```python
from build123d import *

# Parameters (mm, degrees)
SKETCH2_R          = 2
CUT_EXTRUDE1_DEPTH = 20.646882704


with BuildPart() as part:
    # Sketch1 → Revolve1 (revolve)
    with BuildSketch(Plane.XY, mode=Mode.PRIVATE) as revolve1_sk:
        Polygon((-4, 0), (-11, 0), (-11, 3), (-5, 3), (-5, 15), (-4, 15), align=None)
    revolve(revolve1_sk.sketch.rotate(Axis((0, -177.201778129, 0), (0, 1, 0)), 180), axis=Axis((0, -177.201778129, 0), (0, 1, 0)))

    # Sketch2 → Cut-Extrude1 (cut, through all)
    with BuildSketch(Plane(origin=(0, 3, 0), x_dir=(1, 0, 0), z_dir=(0, 1, 0))):
        with Locations(Location((0, 8, 0), (0, 0, 180))):
            Circle(SKETCH2_R)
        with Locations(Location((8, 0, 0), (0, 0, 180))):
            Circle(SKETCH2_R)
        with Locations(Location((0, -8, 0), (0, 0, 180))):
            Circle(SKETCH2_R)
        with Locations(Location((-8, 0, 0), (0, 0, 180))):
            Circle(SKETCH2_R)
    extrude(amount=-CUT_EXTRUDE1_DEPTH, mode=Mode.SUBTRACT)


solid = part.part
```
Source: CAD feature listing. Evaluate the final solid. Frame: model axes, mm. A direction names the side the tool comes from. Coordinates: 2 decimals unless noted, no trailing zeros. Order: outer loops, then holes, each group sorted by start corner. A loop starts at its lowest first (then second) coordinate and runs counter-clockwise, first axis right, second up. Notation, with made-up numbers: (-29.75, 81) - (-15.75, 81) arc R15 cw to (-15.75, 108) - close; hole circle Ø3 at (-4.75, 5). An arc over 180 degrees is marked (long way). One line per item, written item: value.
1) Cut plane D-D on z = -8. Output: boundary loops of the cut face in (x, y), plus the area to 3 significant figures.
Computed values:
outline: (-7.55, 0) - (-2, 0) - (-2, 3) - (-7.55, 3) - close; (2, 0) - (7.55, 0) - (7.55, 3) - (2, 3) - close
area: 33.3 mm^2
2) Contact query for flat-ended pins moving along their axis: pin 1 (4 mm diameter, centred on x = 6, z = -4, fed in from -Y); pin 2 (5 mm diameter, centred on x = -8, z = 0, fed in from +Y); pin 3 (5 mm diameter, centred on x = -3.5, y = 3, fed in from +Z); pin 4 (8 mm diameter, centred on x = -7.5, y = 9, fed in from -Z). Output: stop coordinate, or through.
Computed values:
pin 1: stops at y = 0
pin 2: stops at y = 3
pin 3: stops at z = 10.95
pin 4: stops at z = -3.57
3) Cut plane C-C on y = 13. Output: boundary loops of the cut face in (x, z).
Computed values:
outline: circle Ø10 at (0, 0); hole circle Ø8 at (0, 0)
4) Reachability of faces 4 (the face through (2, 3, 5)), 5 (the face through (-2.38, 1.52, 10.74)) from +Z, -Z, +X, -X, +Y, -Y: full face, straight path, thin tool, end or side. Return the list, or none.
Computed values:
face 4: +Y
face 5: +Y, -Y
5) Ray query, line 1 (X direction, y = 1.75, z = 0.75); line 2 (Y direction, x = -3, z = -7.5); line 3 (Z direction, x = 1.5, y = 0.5). Return the intervals inside material, ascending. Write a range as [from, to].
Computed values:
line 1: x = [-10.97, -9.85], [-6.15, -3.93], [3.93, 6.15], [9.85, 10.97]
line 2: y = [0, 3]
line 3: z = [-10.9, -9.32], [-6.68, -3.71], [3.71, 6.68], [9.32, 10.9]
6) Cut plane A-A on z = 3. Output: boundary loops of the cut face in (x, y).
Computed values:
outline: (-10.58, 0) - (-2.65, 0) - (-2.65, 15) - (-4, 15) - (-4, 3) - (-10.58, 3) - close; (2.65, 0) - (10.58, 0) - (10.58, 3) - (4, 3) - (4, 15) - (2.65, 15) - close
7) Mould query, pull axis Z, two halves, no side actions, for faces 1 (the face through (9.6, 1.5, -1.2)), 2 (the face through (0, 0, 5)), 3 (the face through (-5, 9, 0)). Classes: released by +Z, released by -Z, zero draft, split by the parting line, or undercut.
Computed values:
face 1: undercut
face 2: zero draft
face 3: split by the parting line
8) Cut plane B-B on x = -9.5. Output: boundary loops of the cut face in (y, z).
Computed values:
outline: (0, -5.55) - (3, -5.55) - (3, -1.32) - (0, -1.32) - close; (0, 1.32) - (3, 1.32) - (3, 5.55) - (0, 5.55) - close
